from build123d import *

# Parameters (mm, degrees)
F0_R     = 10
F0_R_2   = 15
F1_DEPTH = 15


with BuildPart() as f1:
    # F0 (on Front) → F1 (new body)
    with BuildSketch(Plane.XZ):
        with BuildLine():
            ThreePointArc((92.840909, 453.603581), (42.840909, 503.603581), (-7.159091, 453.603581))
            Line((-7.159091, 453.603581), (-7.159091, -196.396419))
            ThreePointArc((-7.159091, -196.396419), (42.840909, -246.396419), (92.840909, -196.396419))
            Line((92.840909, -196.396419), (92.840909, 453.603581))
        make_face()
        with Locations((42.840909, -196.396419)):
            Circle(F0_R, mode=Mode.SUBTRACT)
        with Locations((43.185845, 453.461479)):
            Circle(F0_R_2, mode=Mode.SUBTRACT)
    extrude(amount=F1_DEPTH)


solid = f1.part
CAD build for the part. Positions are in the model's coordinates, mm. Give positions to 0.01 mm unless a question says otherwise; leave off trailing zeros. Order: outer loops, then holes, each group sorted by start corner. A loop starts at its lowest first (then second) coordinate and runs counter-clockwise, first axis right, second up. Notation, with made-up numbers: (-39.75, -2) -> (19.25, -2) arc R26 cw to (19.25, 23) -> close; hole circle Ø8 at (-24.5, 27). An arc over 180 degrees is marked (long way). Return JSON: item names as keys, results as strings.
Q1. Mould opens along X. For faces 1 (the face through (39.93, -7.4, 438.82)), 2 (the face through (42, -15, 134)), 3 (the face through (-7.159, -7, 133)), 4 (the face through (40.673, -7.395, -206.159)) say: pulls with the +X half, pulls with the -X half, needs draft (parallel to the pull), parting line crosses it, or undercut.
Working result:
{"face 1": "undercut", "face 2": "needs draft", "face 3": "pulls with the -X half", "face 4": "undercut"}
Q2. Saw through at B-B (x = 75). Write the cut outline in (y, z).
Working result:
{"outline": "(-15, -234.68) -> (0, -234.68) -> (0, 491.89) -> (-15, 491.89) -> close"}
Q3. Drill centre lines: line 1 (Z direction, x = 51.5, y = -0.75); line 2 (Z direction, x = 3, y = -11.75); line 3 (Z direction, x = 71, y = -10.75). Where is each one in solid material? Low to high.
Working result:
{"line 1": "-245.64 to -201.4, -191.39 to 440.98, 465.95 to 502.85", "line 2": "-226.61 to 483.81", "line 3": "-237.71 to 494.92"}
Q4. Saw through at A-A (y = -8.5). Write the cut outline in (x, z).
Working result:
{"outline": "(-7.16, -196.4) arc R50 ccw to (92.84, -196.4) -> (92.84, 453.6) arc R50 ccw to (-7.16, 453.6) -> close; hole circle Ø30 at (43.19, 453.46); hole circle Ø20 at (42.84, -196.4)"}
Q5. Saw through at C-C (x = 7). Write the cut outline in (y, z), then the cut area to 3 significant figures.
Working result:
{"outline": "(-15, -231.26) -> (0, -231.26) -> (0, 488.47) -> (-15, 488.47) -> close", "area": "10,800 mm²"}
Q6. Flat gauge pins, fed straight in: pin 1 (5 mm diameter, centred on x = 68, z = 321, fed in from +Y); pin 2 (1 mm diameter, centred on x = 75, y = -11, fed in from +Z); pin 3 (18 mm diameter, centred on x = 42.84, z = -196.4, fed in from -Y); pin 4 (6 mm diameter, centred on x = 28, y = -2.5, fed in from -Z). Where does each tip first touch, or does it go through?
Working result:
{"pin 1": "y = 0", "pin 2": "z = 492.3", "pin 3": "through", "pin 4": "z = -244.97"}
